from build123d import *

# Parameters (mm, degrees)
SKETCH1_R               = 37.5
BOSS_EXTRUDE1_DEPTH     = 40
SKETCH2_R               = 42.5
BOSS_EXTRUDE2_DEPTH     = 10
CUT_EXTRUDE1_DEPTH      = 40
CUT_EXTRUDE1_DEPTH_BACK = 10
SKETCH3_R               = 27.5


with BuildPart() as part:
    # Sketch1 → Boss-Extrude1 (new body)
    with BuildSketch(Plane(origin=(0, 0, 0), x_dir=(1, 0, 0), z_dir=(0, 1, 0))):
        with Locations(Location((0, 0, 0), (0, 0, 270))):
            Circle(SKETCH1_R)
    extrude(amount=BOSS_EXTRUDE1_DEPTH)

    # Sketch2 → Boss-Extrude2 (add)
    with BuildSketch(Plane(origin=(0, 0, 0), x_dir=(1, 0, 0), z_dir=(0, 1, 0))):
        with Locations(Location((0, 0, 0), (0, 0, 270))):
            Circle(SKETCH2_R)
    extrude(amount=-BOSS_EXTRUDE2_DEPTH)

    # Sketch3 → Cut-Extrude1 (cut, two sides: drawn at the far end of the back side and taken through both)
    with BuildSketch(Plane(origin=(0, 0, 0), x_dir=(1, 0, 0), z_dir=(0, 1, 0)).offset(-CUT_EXTRUDE1_DEPTH_BACK)):
        with Locations(Location((0, 0, 0), (0, 0, 270))):
            Circle(SKETCH3_R)
    extrude(amount=CUT_EXTRUDE1_DEPTH + CUT_EXTRUDE1_DEPTH_BACK, mode=Mode.SUBTRACT)

    # Sketch12 → CBORE for #4 Binding Head Machine Screw1 (revolve, cut)
    with BuildSketch(Plane(origin=(38, 21.382704805, 0), x_dir=(0, 0, -1), z_dir=(0, 1, 0))):
        Polygon((0, 0), (0, 18.885187864), (1.4732, 18), (1.4732, 1.7272), (3.37312, 1.7272), (3.37312, 0.624012762), (4.00812, 0), align=None)
    revolve(axis=Axis((44.35, 21.382704805, 0), (-1, 0, 0)), mode=Mode.SUBTRACT)


solid = part.part
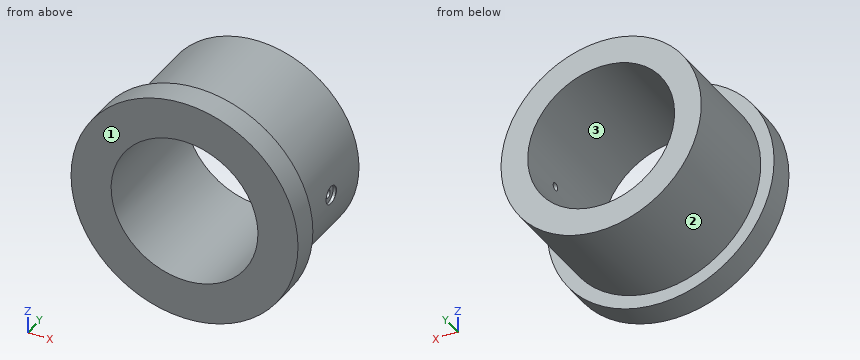
Here's how the part is built. I have some questions about the finished solid (model axes, mm). Face numbers are marked on the shaded views. Coordinates: 2 decimals unless noted, no trailing zeros. Write each loop counter-clockwise with the first axis right and the second up, starting at its lowest first coordinate (ties: lowest second). Pieces come first, ordered by that corner, then holes.
Item 1: Will these pins go through, and if not, where does the flat tip stop? pin 1 (8 mm diameter, centred on y = 21.38, z = 0, fed in from +X); pin 2 (8 mm diameter, centred on x = 32, y = 11.5, fed in from -Z); pin 3 (1 mm diameter, centred on x = -12, y = -4, fed in from -Z).
Item 2: I want a section at C-C on y = 29.5. Write out the boundary of the cut face in (x, z), and give its area (3 significant figures).
Item 3: I want a section at D-D on z = 23. Write out the boundary of the cut face in (x, y), and give its area (3 significant figures).
Item 4: If we mould it in two halves opening along X, with no side actions, what happens to the marked faces 1, 2 and 3? For each: +X half, -X half, draft (parallel to the pull), parting line (faces both ways), or undercut.
Item 5: I want a section at B-B on x = 0. Write out the boundary of the cut face in (y, z).
Item 6: If I drill on line 1 (X direction, y = -0.5, z = 0); line 2 (X direction, y = 7, z = 0); line 3 (Y direction, x = 32, z = 0), over which ranges is the centre line in solid material (lowest first)?
Item 7: I want a section at A-A on z = 0. Write out the boundary of the cut face in (x, y).
Findings below:
1. pin 1: stops at x = 37.5
1. pin 2: stops at z = -24.94
1. pin 3: stops at z = -40.91
2. outline: circle Ø75 at (0, 0); hole circle Ø55 at (0, 0)
2. area: 2,040 mm2
3. outline: (-35.74, -10) - (-15.07, -10) - (-15.07, 40) - (-29.62, 40) - (-29.62, 0) - (-35.74, 0) - close; (15.07, -10) - (35.74, -10) - (35.74, 0) - (29.62, 0) - (29.62, 40) - (15.07, 40) - close
3. area: 1,580 mm2
4. face 1: draft
4. face 2: parting line
4. face 3: undercut
5. outline: (-10, -42.5) - (0, -42.5) - (0, -37.5) - (40, -37.5) - (40, -27.5) - (-10, -27.5) - close; (-10, 27.5) - (40, 27.5) - (40, 37.5) - (0, 37.5) - (0, 42.5) - (-10, 42.5) - close
6. line 1: x = -42.5 to -27.5, 27.5 to 42.5
6. line 2: x = -37.5 to -27.5, 27.5 to 37.5
6. line 3: y = -10 to 19.91, 22.86 to 40
7. outline: (-42.5, -10) - (-27.5, -10) - (-27.5, 40) - (-37.5, 40) - (-37.5, 0) - (-42.5, 0) - close; (27.5, -10) - (42.5, -10) - (42.5, 0) - (37.5, 0) - (37.5, 17.88) - (37.38, 18.01) - (36.27, 18.01) - (36.27, 19.91) - (27.5, 19.91) - close; (27.5, 22.86) - (36.27, 22.86) - (36.27, 24.76) - (37.38, 24.76) - (37.5, 24.88) - (37.5, 40) - (27.5, 40) - close
